Geometry check sheet. Reference: the model listing, model coordinates, mm. Coordinates: 2 decimals unless noted, no trailing zeros. Loops run counter-clockwise (first coordinate to the right, second up) from the corner with the lowest first, then second, coordinate; pieces in that order, holes last. Notation, with made-up numbers: (54, -26) - (84, -26) arc R23 ccw to (84, 5) - close; hole circle Ø7 at (24, 81). An arc over 180 degrees is marked (long way). One line per item, written item: value.
from build123d import *

# Parameters (mm, degrees)
SKETCH1_R               = 70
SKETCH1_R_2             = 12.7
BOSS_EXTRUDE1_DEPTH     = 5
CUT_EXTRUDE1_DEPTH      = 100.121138008
CUT_EXTRUDE1_DEPTH_BACK = 100.121138008
SKETCH3_R               = 2.778125


with BuildPart() as part:
    # Sketch1 → Boss-Extrude1 (new body)
    with BuildSketch(Plane.XY):
        Circle(SKETCH1_R)
        Circle(SKETCH1_R_2, mode=Mode.SUBTRACT)
    extrude(amount=BOSS_EXTRUDE1_DEPTH)

    # Sketch3 → Cut-Extrude1 (cut, two sides: drawn at the far end of the back side and taken through both)
    with BuildSketch(Plane.XY.offset(5).offset(-CUT_EXTRUDE1_DEPTH_BACK)):
        with Locations((-9.5170625, 16.484035789)):
            Circle(SKETCH3_R)
        with Locations((19.034125, 0)):
            Circle(SKETCH3_R)
        with Locations((-9.5170625, -16.484035789)):
            Circle(SKETCH3_R)
    extrude(amount=CUT_EXTRUDE1_DEPTH + CUT_EXTRUDE1_DEPTH_BACK, mode=Mode.SUBTRACT)


solid = part.part
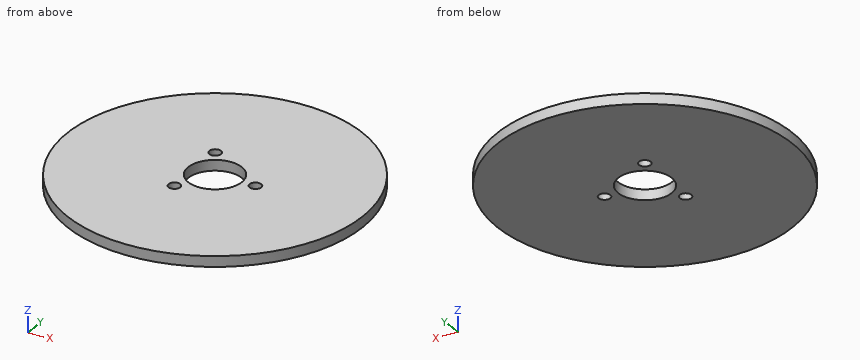
(1) Cross-section at B-B on x = 0. Record the cut outline in (y, z), and give its area (3 significant figures).
Reply:
outline: (-70, 0) - (-12.7, 0) - (-12.7, 5) - (-70, 5) - close; (12.7, 0) - (70, 0) - (70, 5) - (12.7, 5) - close
area: 573 mm2
(2) Material ranges on probe 1 along Y at (x, z) = (1, 0.7); probe 2 along X at (y, z) = (-11, 4.5); probe 3 along Y at (x, z) = (-11, 3.05), recorded low to high. Write a range as from..to.
Reply:
probe 1: -69.99..-12.66, 12.66..69.99
probe 2: -69.13..-6.35, 6.35..69.13
probe 3: -69.13..-18.83, -14.13..-6.35, 6.35..14.13, 18.83..69.13
(3) Go/stop test with flat-tipped pins: pin 1 Ø1 at (y, z) = (-31, 3.5) entering from +X; pin 2 Ø3 at (x, z) = (27, 3) entering from +Y; pin 3 Ø3 at (y, z) = (20, 1) entering from -X. Record where each tip stops, or that it passes through.
Reply:
pin 1: x = 63.01
pin 2: y = 65.19
pin 3: x = -67.51
(4) Cross-section at A-A on y = 0. Record the cut outline in (x, z), and give its area (3 significant figures).
Reply:
outline: (-70, 0) - (-12.7, 0) - (-12.7, 5) - (-70, 5) - close; (12.7, 0) - (16.26, 0) - (16.26, 5) - (12.7, 5) - close; (21.81, 0) - (70, 0) - (70, 5) - (21.81, 5) - close
area: 545 mm2
(5) Cross-section at D-D on x = -28. Record the cut outline in (y, z), and give its area (3 significant figures).
Reply:
outline: (-64.16, 0) - (64.16, 0) - (64.16, 5) - (-64.16, 5) - close
area: 642 mm2
(6) Cross-section at C-C on z = 1.5. Record the cut outline in (x, y).
Reply:
outline: circle Ø140 at (0, 0); hole circle Ø25.4 at (0, 0); hole circle Ø5.56 at (-9.52, -16.48); hole circle Ø5.56 at (-9.52, 16.48); hole circle Ø5.56 at (19.03, 0)
